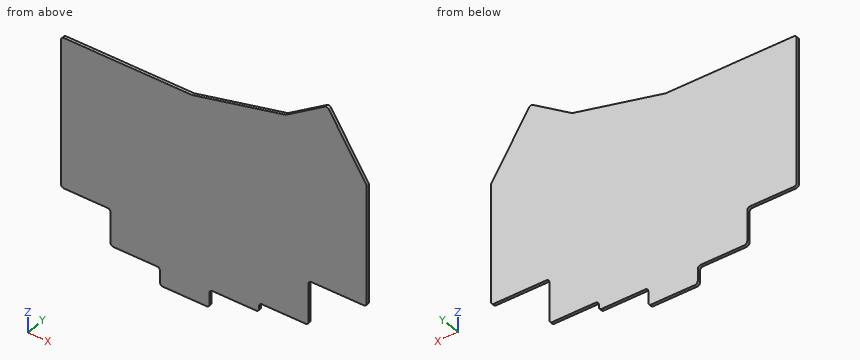
```python
from build123d import *

# Parameters (mm, degrees)
RESSALTO_EXTRUS_O1_DEPTH = 1
FILETE1_R                = 1


with BuildPart() as part:
    # Esboço1 → Ressalto-extrusão1 (new body)
    with BuildSketch(Plane(origin=(0, 0, 0), x_dir=(1, 0, 0), z_dir=(0, 1, 0))):
        Polygon((-58.0333979, 11.326122728), (-58.0333979, 62.326122728), (-41.0333979, 62.326122728), (-41.0333979, 74.689759091), (-24.0333979, 74.689759091), (-24.0333979, 80.689759091), (-7.0333979, 80.689759091), (-7.0333979, 74.689759091), (9.9666021, 74.689759091), (9.9666021, 71.689759091), (26.9666021, 71.689759091), (26.9666021, 56.689759091), (46.9666021, 56.689759091), (46.9666021, 15.689759091), (33.403566363, -5.311289968), (19.122853002, 3.911574333), (-13.0333979, 11.326122728), align=None)
    extrude(amount=RESSALTO_EXTRUS_O1_DEPTH)

    # Filete1
    filete1_edges = [part.edges().sort_by_distance(p)[0] for p in [
        (-58.0333979, 0.5, -11.326122728),
        (-58.0333979, 0.5, -62.326122728),
        (-41.0333979, 0.5, -62.326122728),
        (-41.0333979, 0.5, -74.689759091),
        (-24.0333979, 0.5, -74.689759091),
        (-24.0333979, 0.5, -80.689759091),
        (-7.0333979, 0.5, -80.689759091),
        (-7.0333979, 0.5, -74.689759091),
        (9.9666021, 0.5, -74.689759091),
        (9.9666021, 0.5, -71.689759091),
        (26.9666021, 0.5, -71.689759091),
        (26.9666021, 0.5, -56.689759091),
        (46.9666021, 0.5, -56.689759091),
        (46.9666021, 0.5, -15.689759091),
        (33.403566363, 0.5, 5.311289968),
        (19.122853002, 0.5, -3.911574333),
        (-13.0333979, 0.5, -11.326122728),
    ]]
    fillet(filete1_edges, radius=FILETE1_R)


solid = part.part
```
Model file for the job. Use its own axes, mm. Round coordinates to 2 decimals unless told otherwise and drop trailing zeros. Write each loop counter-clockwise with the first axis right and the second up, starting at its lowest first coordinate (ties: lowest second). Pieces come first, ordered by that corner, then holes. Notation, with made-up numbers: (58, 49) - (93, 49) arc R23 ccw to (93, 61) - close; hole circle Ø2 at (-13, 89). An arc over 180 degrees is marked (long way). Use CSV: the item, a comma, the result in double quotes. Start each with the question number.
Item 1: Drill centre lines: L1, parallel to Z at x = -43, y = 0.6; L2, parallel to Z at x = -29.5, y = 0.85; L3, parallel to X at y = 0.15, z = -66.5. Where is each one in solid material? Low to high. Write a range as [from, to].
Item 2: Band-saw the part on C-C (z = -69.5). Write the cut outline in (x, y), and give its area (3 significant figures).
Item 3: Pin check, flat tips, straight feed: P1, Ø0.5, axis at y = 0.5, z = -65, coming from the +X side; P2, Ø0.5, axis at x = 16.5, y = 0.5, coming from the -Z side; P3, Ø0.5, axis at y = 0.5, z = -78, coming from the +X side. Stop position of each tip, or through.
Item 4: Band-saw the part on B-B (x = -18.5). Write the cut outline in (y, z), and give its area (3 significant figures).
Checked values:
1,L1,"z = [-62.33, -11.33]"
1,L2,"z = [-74.69, -11.33]"
1,L3,"x = [-41.03, 26.97]"
2,outline,"(-41.03, 0) - (26.97, 0) - (26.97, 1) - (-41.03, 1) - close"
2,area,"68.0 mm²"
3,P1,"stops at x = 26.97"
3,P2,"stops at z = -71.69"
3,P3,"stops at x = -7.03"
4,outline,"(0, -80.69) - (1, -80.69) - (1, -11.33) - (0, -11.33) - close"
4,area,"69.4 mm²"
